Build history of the part. All positions in model axes, mm. Face numbers are marked on the shaded views. A direction names the side the tool comes from. Coordinates: 2 decimals unless noted, no trailing zeros. Write each loop counter-clockwise with the first axis right and the second up, starting at its lowest first coordinate (ties: lowest second). Pieces come first, ordered by that corner, then holes. Notation, with made-up numbers: M 30,0.25 L 35,0.25 A25 ccw 35,21.25 Z; hole C -32,87.25 d4. An arc over 180 degrees is marked long. Use CSV: the item, a comma, the result in double quotes. Start each with the question number.
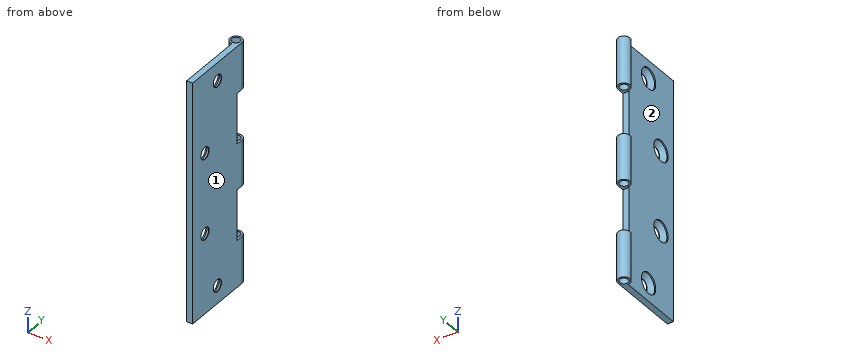
```python
from build123d import *

# Parameters (mm, degrees)
SKETCH1_W                                      = 5
SKETCH1_H                                      = 60
EXTRUDE_THIN1_DEPTH                            = 100
SKETCH2_R                                      = 5
SKETCH3_R                                      = 3.5
CUT_EXTRUDE1_DEPTH                             = 211.35683968
CSK_FOR_M8_FLAT_HEAD_MACHINE_SCREW1_AT_2_COUNT = 2
CSK_FOR_M8_FLAT_HEAD_MACHINE_SCREW1_AT_2_PITCH = 53.800041305
F_2_CUTS_DEPTH                                 = 120.373363863
F_2_CUTS_DEPTH_BACK                            = 120.373363863
SKETCH8_W                                      = 42
SKETCH8_H                                      = 11


with BuildPart() as part:
    # Sketch1 → Extrude-Thin1 (new, symmetric)
    with BuildSketch(Plane.XY):
        with Locations((2.5, 30)):
            Rectangle(SKETCH1_W, SKETCH1_H)
    extrude(amount=EXTRUDE_THIN1_DEPTH, both=True)

    # Sweep1: sweep along a curve in space
    with BuildLine() as sweep1_path:
        Line((0, 60, 100), (0, 60, -100))
    # Sketch2 → Sweep1 (sweep)
    with BuildSketch(Plane(origin=(0, 0, -100), x_dir=(-1, 0, 0), z_dir=(0, 0, -1))):
        with Locations((0, 60)):
            Circle(SKETCH2_R)
    sweep(path=sweep1_path.line)

    # Sketch3 → Cut-Extrude1 (cut, through all)
    with BuildSketch(Plane(origin=(0, 0, -100), x_dir=(-1, 0, 0), z_dir=(0, 0, -1))):
        with Locations((0, 60)):
            Circle(SKETCH3_R)
    extrude(amount=-CUT_EXTRUDE1_DEPTH, mode=Mode.SUBTRACT)

    # Sketch4 → CSK for M8 Flat Head Machine Screw1 (revolve, cut)
    with BuildSketch(Plane(origin=(0, 30, -85), x_dir=(0, 0, 1), z_dir=(0, 1, 0))):
        Polygon((0, 0), (0, 5), (5, 5), (5, 4.65), (8.65, 1), (8.65, 0), align=None)
    csk_for_m8_flat_head_machine_screw1 = revolve(axis=Axis((-6.35, 30, -85), (1, 0, 0)), mode=Mode.SUBTRACT)

    # CSK for M8 Flat Head Machine Screw1 at 2: CSK for M8 Flat Head Machine Screw1 ×2
    with Locations(*[Vector(0, -0.2788101948639552, 0.9603462267536241) * (i * CSK_FOR_M8_FLAT_HEAD_MACHINE_SCREW1_AT_2_PITCH) for i in range(1, CSK_FOR_M8_FLAT_HEAD_MACHINE_SCREW1_AT_2_COUNT)]):
        add(csk_for_m8_flat_head_machine_screw1, mode=Mode.SUBTRACT)

    # Mirror1: CSK for M8 Flat Head Machine Screw1 across plane
    add(csk_for_m8_flat_head_machine_screw1.mirror(Plane.XY), mode=Mode.SUBTRACT)

    # Mirror1 copy 1 sketch → Mirror1 copy 1 (revolve, cut)
    with BuildSketch(Plane(origin=(0, 15, 33.333333333), x_dir=(0, 0, -1), z_dir=(0, 1, 0))):
        Polygon((0, 0), (0, -5), (5, -5), (5, -4.65), (8.65, -1), (8.65, 0), align=None)
    revolve(axis=Axis((-6.35, 15, 33.333333333), (-1, 0, 0)), mode=Mode.SUBTRACT)

    # Sketch8 → 2 cuts (cut, two sides: drawn at the far end of the back side and taken through both)
    with BuildSketch(Plane.ZY.offset(-F_2_CUTS_DEPTH_BACK)):
        with Locations((-40, 59.5)):
            Rectangle(SKETCH8_W, SKETCH8_H)
        with Locations((40, 59.5)):
            Rectangle(SKETCH8_W, SKETCH8_H)
    extrude(amount=F_2_CUTS_DEPTH + F_2_CUTS_DEPTH_BACK, mode=Mode.SUBTRACT)


solid = part.part
```
1. 3-axis set-ups, long thin cutter, end or side, ignore diameter. For the marked faces 1 and 2: which of +Z, -Z, +X, -X, +Y, -Y reach the whole face in a straight line?
2. Slice it at C-C (y = 51.5). List the corners of the cut face in (x, z).
3. Drill centre lines: line 1 along Z through (x, y) = (0.5, 30); line 2 along Y through (x, z) = (0.3, -85); line 3 along Z through (x, y) = (4.8, 30). Where is each one in solid material? Low to high. Write a range as from..to.
4. Slice it at A-A (y = 15). List the corners of the cut face in (x, z).
5. Slice it at B-B (x = -1.5). List the corners of the cut face in (y, z).
6. Flat gauge pins, fed straight in: pin 1 (8 mm diameter, centred on y = 29, z = 1, fed in from -X); pin 2 (10.5 mm diameter, centred on y = 30, z = -85, fed in from -X); pin 3 (1.5 mm diameter, centred on x = 1.5, z = 33, fed in from +Y). Where does each tip first touch, or does it go through?
7. Slice it at D-D (y = 27). Count the separate pieces of the cut face and the enclosed holes in it, and give its area (3 significant figures).
Established:
1,face 1,"+Z, -Z, +X, +Y, -Y"
1,face 2,"+Z, -Z, -X, -Y"
2,outline,"M 0,-100 L 5,-100 L 5,100 L 0,100 Z"
3,line 1,"z = -100..-93.65, -76.35..76.35, 93.65..100"
3,line 2,"y = 0..21.35, 38.65..56.51, 63.49..64.99"
3,line 3,"z = -100..-90, -80..80, 90..100"
4,outline,"M 0,-100 L 5,-100 L 5,-38.33 L 4.65,-38.33 L 1,-41.98 L 0,-41.98 Z; M 0,-24.68 L 1,-24.68 L 4.65,-28.33 L 5,-28.33 L 5,28.33 L 4.65,28.33 L 1,24.68 L 0,24.68 Z; M 0,41.98 L 1,41.98 L 4.65,38.33 L 5,38.33 L 5,100 L 0,100 Z"
5,outline,"M 55.23,-100 L 56.84,-100 L 56.84,-61 L 55.23,-61 Z; M 55.23,-19 L 56.84,-19 L 56.84,19 L 55.23,19 Z; M 55.23,61 L 56.84,61 L 56.84,100 L 55.23,100 Z; M 63.16,-100 L 64.77,-100 L 64.77,-61 L 63.16,-61 Z; M 63.16,-19 L 64.77,-19 L 64.77,19 L 63.16,19 Z; M 63.16,61 L 64.77,61 L 64.77,100 L 63.16,100 Z"
6,pin 1,"stops at x = 0"
6,pin 2,"stops at x = 4.4"
6,pin 3,"stops at y = 54"
7,separate pieces,"3"
7,enclosed holes,"0"
7,area,"873 mm2"
